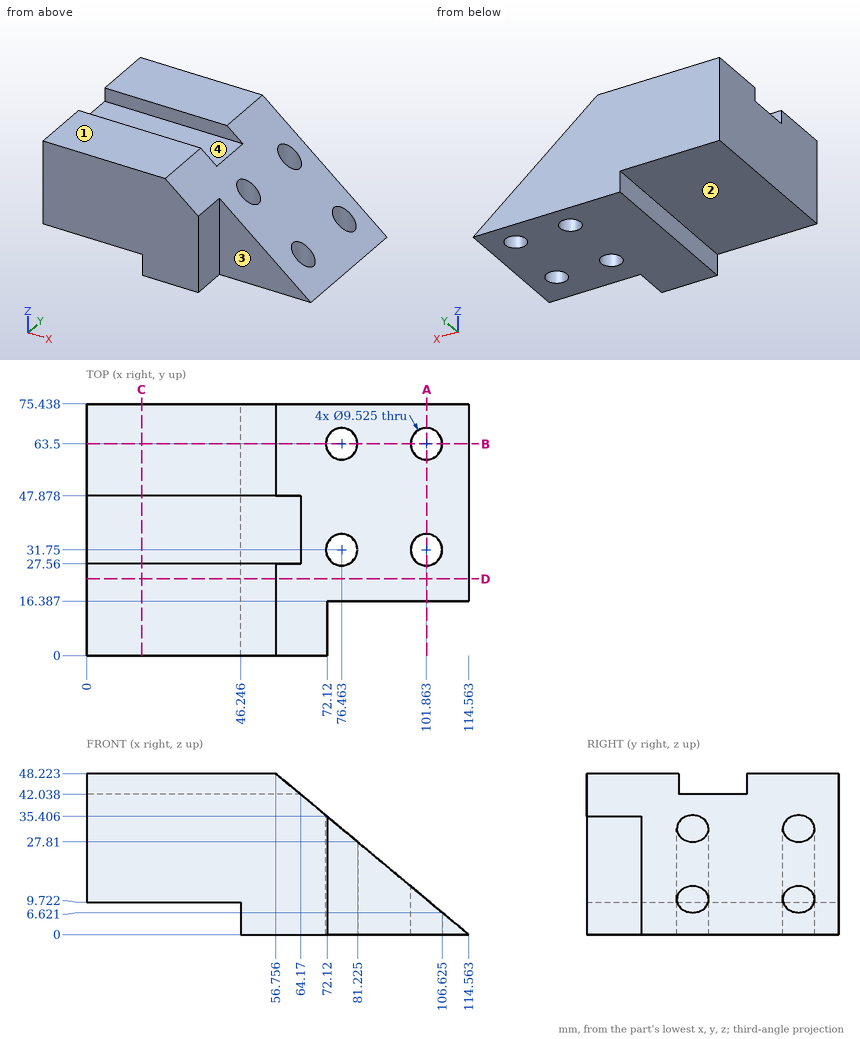
Check sheet for the drawn part. Datum: minimum x, y, z corner. Units: mm. A direction names the side the tool comes from. Round coordinates to 2 decimals unless told otherwise and drop trailing zeros. Write each loop counter-clockwise with the first axis right and the second up, starting at its lowest first coordinate (ties: lowest second). Pieces come first, ordered by that corner, then holes. Notation, with made-up numbers: (-37, 43.5) -> (-32, 43.5) arc R28 cw to (-32, 78.5) -> close; hole circle Ø8 at (-11, 50.25). An arc over 180 degrees is marked (long way). Write each question's results on one line, items separated by ' | '. Start each with the question number.
1. Cross-section at D-D (y = 23). Enter the section's corners in (x, z) (1 decimal), then the cut area to 3 significant figures.
2. Set-up check for the marked faces 1, 2, 3 and 4: record each of +Z, -Z, +X, -X, +Y, -Y from which the full face is reachable in a straight line by a thin tool's end or side.
3. Material ranges on probe 1 along Y at (x, z) = (79.5, 14.5) (1 decimal); probe 2 along X at (y, z) = (63.5, 9.5) (1 decimal); probe 3 along X at (y, z) = (31.75, 4.5) (1 decimal), recorded low to high. Write a range as from..to.
4. Cross-section at B-B (y = 63.5). Enter the section's corners in (x, z) (1 decimal), then the cut area to 3 significant figures.
5. Cross-section at A-A (x = 102). Enter the section's corners in (y, z), then the cut area to 3 significant figures.
6. Cross-section at C-C (x = 16.5). Enter the section's corners in (y, z).
7. Depth check by flat-ended pin: P1, Ø16.5, axis at x = 16.5, y = 39.5, coming from the +Z side; P2, Ø8, axis at y = 5, z = 10.5, coming from the +X side; P3, Ø5.5, axis at x = 101.86, y = 31.75, coming from the +Z side; P4, Ø3, axis at y = 23, z = 6.5, coming from the -X side. Enter the tip coordinate at first touch or a pass-through.
Solutions:
1) outline: (0, 9.7) -> (46.2, 9.7) -> (46.2, 0) -> (114.6, 0) -> (56.8, 48.2) -> (0, 48.2) -> close | area: 3,680 mm2
2) face 1: +Z, +X, -X, +Y, -Y | face 2: -Z, -X, +Y, -Y | face 3: +Z, -Z, +X, -Y | face 4: +Z, +X, -X
3) probe 1: y = 16.4..28.1, 35.4..59.8, 67.2..75.4 | probe 2: x = 46.2..71.7, 81.2..97.1 | probe 3: x = 46.2..71.7, 81.2..97.1, 106.6..109.2
4) outline: (0, 9.7) -> (46.2, 9.7) -> (46.2, 0) -> (71.7, 0) -> (71.7, 35.8) -> (56.8, 48.2) -> (0, 48.2) -> close; (81.2, 0) -> (97.1, 0) -> (97.1, 14.6) -> (81.2, 27.8) -> close; (106.6, 0) -> (114.6, 0) -> (106.6, 6.6) -> close | area: 3,280 mm2
5) outline: (16.39, 0) -> (26.99, 0) -> (26.99, 10.48) -> (16.39, 10.48) -> close; (36.51, 0) -> (58.74, 0) -> (58.74, 10.48) -> (36.51, 10.48) -> close; (68.26, 0) -> (75.44, 0) -> (75.44, 10.48) -> (68.26, 10.48) -> close | area: 419 mm2
6) outline: (0, 9.72) -> (75.44, 9.72) -> (75.44, 48.22) -> (47.88, 48.22) -> (47.88, 42.04) -> (27.56, 42.04) -> (27.56, 48.22) -> (0, 48.22) -> close
7) P1: stops at z = 42.04 | P2: stops at x = 72.12 | P3: passes through | P4: stops at x = 46.25
